CAD build for the part. Positions are in the model's coordinates, mm. Face numbers are marked on the shaded views. A direction names the side the tool comes from. Coordinates: 2 decimals unless noted, no trailing zeros. Loops run counter-clockwise (first coordinate to the right, second up) from the corner with the lowest first, then second, coordinate; pieces in that order, holes last. Notation, with made-up numbers: (42.5, 74) -> (75.5, 74) arc R26 ccw to (75.5, 93) -> close; hole circle Ø8 at (69, 4). An arc over 180 degrees is marked (long way). Return JSON: item names as keys, results as strings. Group by question number.
(1) Flat gauge pins, fed straight in: pin 1 Ø6 at (y, z) = (11.5, 1.5) entering from -X; pin 2 Ø4 at (y, z) = (24.5, -2.5) entering from +X; pin 3 Ø1.5 at (x, z) = (15, 1) entering from -Y. Where does each tip first touch, or does it go through?
(2) Saw through at B-B on x = 14.25. Write the cut outline in (y, z), then the cut area to 3 significant figures.
(3) Saw through at C-C on z = -4.25. Write the cut outline in (x, y).
(4) Saw through at D-D on y = 7. Write the cut outline in (x, z), then the cut area to 3 significant figures.
(5) Saw through at A-A on x = -14.25. Write the cut outline in (y, z), then the cut area to 3 significant figures.
(6) Mould opens along Y. For the marked faces 5, 6 and 7 say: pulls with the +Y half, pulls with the -Y half, needs draft (parallel to the pull), parting line crosses it, or undercut.
(7) Probe L1, parallel to X at y = 18.9, z = 0; L2, parallel to X at y = 29.05, z = 0; L3, parallel to Z at x = -14.25, y = 19.65. List the from-to ranges inside material, lowest first.
(8) Tool access for the marked faces 1, 2, 3 and 4: list every direction of +Z, -Z, +X, -X, +Y, -Y with a clear straight run to the whole face (end or side of a thin tool).
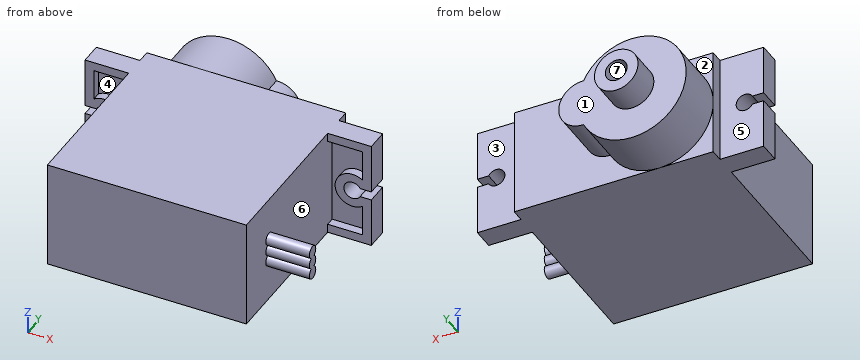
```python
from build123d import *

# Parameters (mm, degrees)
SKETCH1_W           = 22.8
SKETCH1_H           = 12.4
BOSS_EXTRUDE1_DEPTH = 22
BOSS_EXTRUDE3_DEPTH = 6
SKETCH3_R           = 2.5
SKETCH3_R_2         = 1.25
BOSS_EXTRUDE4_DEPTH = 3.5
BOSS_EXTRUDE5_DEPTH = 2.5
CUT_EXTRUDE1_DEPTH  = 1
BOSS_EXTRUDE6_DEPTH = 5


with BuildPart() as part:
    # Sketch1 → Boss-Extrude1 (new body)
    with BuildSketch(Plane(origin=(0, 0, 0), x_dir=(1, 0, 0), z_dir=(0, 1, 0))):
        Rectangle(SKETCH1_W, SKETCH1_H)
    extrude(amount=BOSS_EXTRUDE1_DEPTH)

    # Sketch2 → Boss-Extrude3 (add)
    with BuildSketch(Plane(origin=(0, 22, 0), x_dir=(1, 0, 0), z_dir=(0, 1, 0))):
        with BuildLine():
            ThreePointArc((0.357522124, 2.748444622), (-11.4, 0), (0.357522124, -2.748444622))
            ThreePointArc((0.357522124, -2.748444622), (3.2, 0), (0.357522124, 2.748444622))
        make_face()
    extrude(amount=BOSS_EXTRUDE3_DEPTH)

    # Sketch3 → Boss-Extrude4 (add)
    with BuildSketch(Plane(origin=(0, 28, 0), x_dir=(1, 0, 0), z_dir=(0, 1, 0))):
        with Locations((-5.2, 0)):
            Circle(SKETCH3_R)
        with Locations((-5.2, 0)):
            Circle(SKETCH3_R_2, mode=Mode.SUBTRACT)
    extrude(amount=BOSS_EXTRUDE4_DEPTH)

    # Sketch4 → Boss-Extrude5 (add)
    with BuildSketch(Plane(origin=(0, 18, 0), x_dir=(1, 0, 0), z_dir=(0, 1, 0))):
        with BuildLine():
            Line((-16.4, -0.5), (-16.4, -6.2))
            Line((-16.4, -6.2), (-11.4, -6.2))
            Line((-11.4, -6.2), (-11.4, 6.2))
            Line((-11.4, 6.2), (-16.4, 6.2))
            Line((-16.4, 6.2), (-16.4, 0.5))
            Line((-16.4, 0.5), (-15.116025404, 0.5))
            ThreePointArc((-15.116025404, 0.5), (-13.25, 0), (-15.116025404, -0.5))
            Line((-15.116025404, -0.5), (-16.4, -0.5))
        make_face()
    boss_extrude5 = extrude(amount=BOSS_EXTRUDE5_DEPTH)

    # Sketch5 → Cut-Extrude1 (cut)
    with BuildSketch(Plane.XZ.offset(-18)):
        with BuildLine():
            Line((-11.4, -5.2), (-11.4, 5.2))
            Line((-11.4, 5.2), (-15.4, 5.2))
            Line((-15.4, 5.2), (-15.4, 1.636306817))
            ThreePointArc((-15.4, 1.636306817), (-12.25, 0), (-15.4, -1.636306817))
            Line((-15.4, -1.636306817), (-15.4, -5.2))
            Line((-15.4, -5.2), (-11.4, -5.2))
        make_face()
    cut_extrude1 = extrude(amount=-CUT_EXTRUDE1_DEPTH, mode=Mode.SUBTRACT)

    # Mirror1: Boss-Extrude5, Cut-Extrude1 across plane
    add(boss_extrude5.mirror(Plane(origin=(0, 0, 0), x_dir=(0, 0, 1), z_dir=(1, 0, 0))))
    add(cut_extrude1.mirror(Plane(origin=(0, 0, 0), x_dir=(0, 0, 1), z_dir=(1, 0, 0))), mode=Mode.SUBTRACT)

    # Sketch6 → Boss-Extrude6 (add)
    with BuildSketch(Plane(origin=(11.4, 0, 0), x_dir=(0, 0, -1), z_dir=(1, 0, 0))):
        with BuildLine():
            ThreePointArc((-0.65, 4.740192379), (0, 4.3), (0.65, 4.740192379))
            ThreePointArc((0.65, 4.740192379), (2, 5), (0.65, 5.259807621))
            ThreePointArc((0.65, 5.259807621), (0, 5.7), (-0.65, 5.259807621))
            ThreePointArc((-0.65, 5.259807621), (-2, 5), (-0.65, 4.740192379))
        make_face()
    extrude(amount=BOSS_EXTRUDE6_DEPTH)


solid = part.part
```
Geometry results:
{
 "1": {"pin 1": "x = -11.4", "pin 2": "x = 3.15", "pin 3": "y = 4.3"},
 "2": {"outline": "(4.74, -0.65) arc R0.7 ccw (long way) to (5.26, -0.65) arc R0.7 ccw to (5.26, 0.65) arc R0.7 ccw (long way) to (4.74, 0.65) arc R0.7 ccw to start; (18, -6.2) -> (20.5, -6.2) -> (20.5, -1) -> (18, -1) -> (18, -2) -> (19, -2) -> (19, -5.2) -> (18, -5.2) -> close; (18, 1) -> (20.5, 1) -> (20.5, 6.2) -> (18, 6.2) -> (18, 5.2) -> (19, 5.2) -> (19, 2) -> (18, 2) -> close", "area": "24.1 mm²"},
 "3": {"outline": "(-16.4, 18) -> (-15.4, 18) -> (-15.4, 19) -> (-11.4, 19) -> (-11.4, 0) -> (11.4, 0) -> (11.4, 19) -> (15.4, 19) -> (15.4, 18) -> (16.4, 18) -> (16.4, 20.5) -> (11.4, 20.5) -> (11.4, 22) -> (-0.69, 22) -> (-0.69, 28) -> (-9.71, 28) -> (-9.71, 22) -> (-11.4, 22) -> (-11.4, 20.5) -> (-16.4, 20.5) -> close"},
 "4": {"outline": "(-11.4, -6.2) -> (11.4, -6.2) -> (11.4, 6.2) -> (-11.4, 6.2) -> close", "area": "283 mm²"},
 "5": {"outline": "(18, -6.2) -> (20.5, -6.2) -> (20.5, -1) -> (18, -1) -> (18, -2) -> (19, -2) -> (19, -5.2) -> (18, -5.2) -> close; (18, 1) -> (20.5, 1) -> (20.5, 6.2) -> (18, 6.2) -> (18, 5.2) -> (19, 5.2) -> (19, 2) -> (18, 2) -> close", "area": "19.6 mm²"},
 "6": {"face 5": "pulls with the +Y half", "face 6": "undercut", "face 7": "needs draft"},
 "7": {"L1": "-13.25 to -12.25, -11.4 to 11.4, 12.25 to 13.25", "L2": "-7.7 to -6.45, -3.95 to -2.7", "L3": "-6.2 to -1, 1 to 6.2"},
 "8": {"face 1": "+Y", "face 2": "+Z, -X, +Y", "face 3": "+Z, -Z, +X, +Y", "face 4": "-Y"}
}
